Input: dimensioned drawing with shaded views. Units: mm. Origin: part minimum x, y, z. A direction names the side the tool comes from. Coordinates: 2 decimals unless noted, no trailing zeros. Loops run counter-clockwise (first coordinate to the right, second up) from the corner with the lowest first, then second, coordinate; pieces in that order, holes last.
(1) Section A-A, the plane x = 130. Return loops of the section in (y, z), then the cut area to 3 significant figures.
(2) Line query: L1, parallel to X at y = 3.5, z = 129 (1 decimal); L2, parallel to Z at x = 97.5, y = 16 (1 decimal); L3, parallel to Z at x = 64.5, y = 3 (1 decimal). Output: solid intervals per line, ascending.
(3) Set-up query: the marked faces 4 and 5. Return all of +Z, -Z, +X, -X, +Y, -Y with unobstructed straight access to the full face (end or side cutting, diameter ignored); none if empty.
(4) Mould query, pull axis X, two halves, no side actions, for the marked faces 1, 2 and 3. Classes: released by +X, released by -X, zero draft, split by the parting line, or undercut.
(5) Contact query for flat-ended pins moving along their axis: P1, Ø4, axis at x = 166.5, y = 19, coming from the -Z side (1 decimal); P2, Ø13.5, axis at x = 184.31, z = 24.38, coming from the -Y side; P3, Ø21, axis at x = 61.5, y = 20, coming from the -Z side. Output: stop coordinate, or through.
(6) Section B-B, the plane z = 151. Return loops of the section in (x, y) (1 decimal), then the cut area to 3 significant figures.
(7) Section C-C, the plane y = 14. Give the number of separate pieces and of enclosed holes in the cut face, then the cut area to 3 significant figures.
(8) Section D-D, the plane x = 185. Return loops of the section in (y, z) (1 decimal), then the cut area to 3 significant figures.
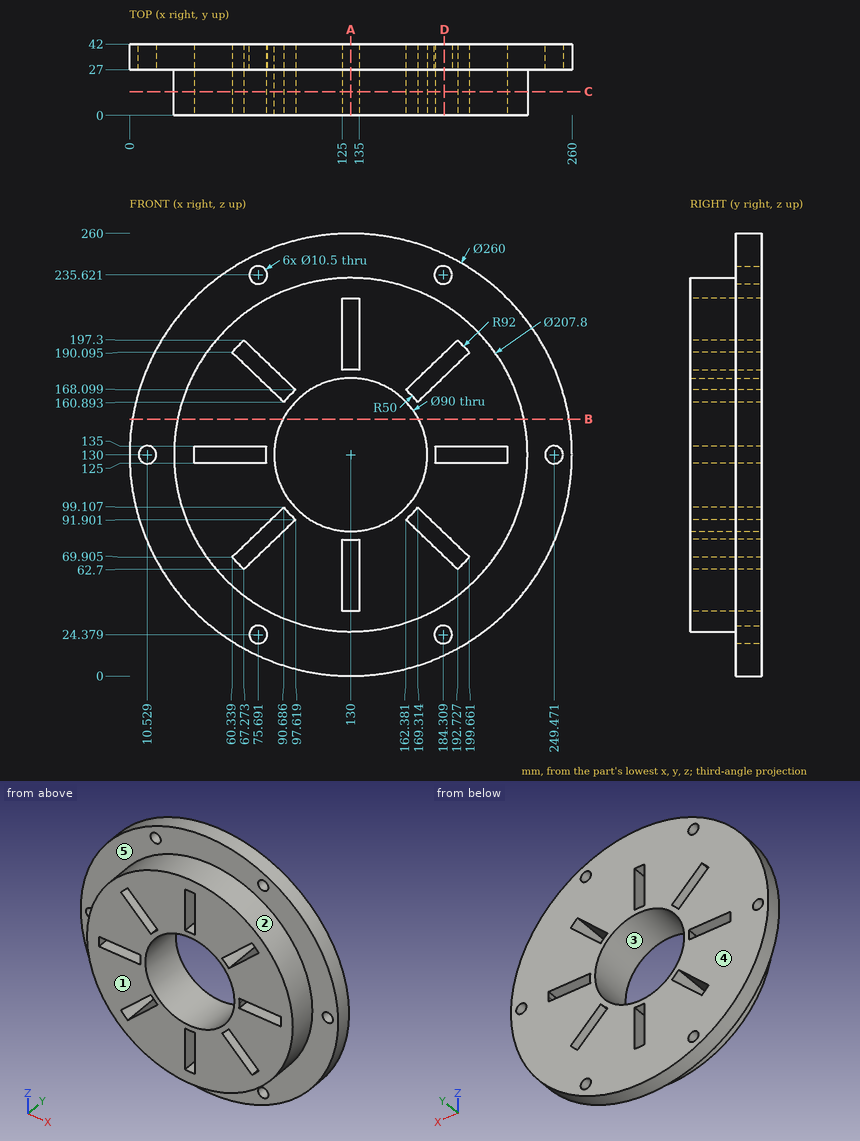
Report:
1. outline: (0, 26.1) - (27, 26.1) - (27, 0) - (42, 0) - (42, 38) - (0, 38) - close; (0, 80) - (42, 80) - (42, 85) - (0, 85) - close; (0, 175) - (42, 175) - (42, 180) - (0, 180) - close; (0, 222) - (42, 222) - (42, 260) - (27, 260) - (27, 233.9) - (0, 233.9) - close
1. area: 2,200 mm2
2. L1: x = 26.1 to 38, 80 to 85, 175 to 180, 222 to 233.9
2. L2: z = 31.3 to 91.8, 92 to 98.9, 161.1 to 168, 168.2 to 228.7
2. L3: z = 49.3 to 65.4, 73.9 to 125, 135 to 186.1, 194.6 to 210.7
3. face 4: +Z, -Z, +X, -X, +Y
3. face 5: -Y
4. face 1: zero draft
4. face 2: split by the parting line
4. face 3: undercut
5. P1: stops at z = 32
5. P2: stops at y = 27
5. P3: stops at z = 15.03
6. outline: (1.7, 27) - (28.2, 27) - (28.2, 0) - (90.2, 0) - (90.2, 42) - (1.7, 42) - close; (169.8, 0) - (231.8, 0) - (231.8, 27) - (258.3, 27) - (258.3, 42) - (169.8, 42) - close
6. area: 6,000 mm2
7. separate pieces: 1
7. enclosed holes: 9
7. area: 24,200 mm2
8. outline: (0, 41.9) - (27, 41.9) - (27, 29.6) - (42, 29.6) - (42, 70.1) - (0, 70.1) - close; (0, 84) - (42, 84) - (42, 125) - (0, 125) - close; (0, 135) - (42, 135) - (42, 176) - (0, 176) - close; (0, 189.9) - (42, 189.9) - (42, 230.4) - (27, 230.4) - (27, 218.1) - (0, 218.1) - close; (27, 12.2) - (42, 12.2) - (42, 19.2) - (27, 19.2) - close; (27, 240.8) - (42, 240.8) - (42, 247.8) - (27, 247.8) - close
8. area: 6,400 mm2
